from build123d import *

# Parameters (mm, degrees)
SKETCH1_W           = 95
SKETCH1_H           = 65
BOSS_EXTRUDE1_DEPTH = 5
FILLET2_R           = 4
SKETCH3_W           = 89.4
SKETCH3_H           = 59.4
BOSS_EXTRUDE3_DEPTH = 3
FILLET3_R           = 4
SHELL1_START        = -3
SHELL1_DEPTH        = 5.5


# Read off the part's stored shape, not the designer's step: Shell1
with BuildPart() as part:
    # Sketch1 → Boss-Extrude1 (new body)
    with BuildSketch(Plane(origin=(0, 0, 0), x_dir=(1, 0, 0), z_dir=(0, 1, 0))):
        with Locations((47.5, 32.5)):
            Rectangle(SKETCH1_W, SKETCH1_H)
    extrude(amount=BOSS_EXTRUDE1_DEPTH)

    # Fillet2
    fillet2_edges = [part.edges().sort_by_distance(p)[0] for p in [
        (95, 5, -32.5),
        (47.5, 5, -65),
        (0, 5, -32.5),
        (0, 2.5, -65),
        (95, 2.5, -65),
        (95, 2.5, 0),
        (0, 2.5, 0),
        (47.5, 5, 0),
    ]]
    fillet(fillet2_edges, radius=FILLET2_R)

    # Sketch3 → Boss-Extrude3 (add)
    with BuildSketch(Plane.XZ):
        with Locations((47.5, -32.5)):
            Rectangle(SKETCH3_W, SKETCH3_H)
    extrude(amount=BOSS_EXTRUDE3_DEPTH)

    # Fillet3
    fillet3_edges = [part.edges().sort_by_distance(p)[0] for p in [
        (2.8, -1.5, -2.8),
        (2.8, -1.5, -62.2),
        (92.2, -1.5, -62.2),
        (92.2, -1.5, -2.8),
    ]]
    fillet(fillet3_edges, radius=FILLET3_R)

    # Shell1 outline → Shell1 (cut)
    with BuildSketch(Plane(origin=(0, 0, 0), x_dir=(1, 0, 0), z_dir=(0, 1, 0)).offset(SHELL1_START)):
        with BuildLine():
            Line((5.3, 58.2), (5.3, 6.8))
            ThreePointArc((5.3, 6.8), (5.739339828, 5.739339828), (6.8, 5.3))
            Line((6.8, 5.3), (88.2, 5.3))
            ThreePointArc((88.2, 5.3), (89.260660172, 5.739339828), (89.7, 6.8))
            Line((89.7, 6.8), (89.7, 58.2))
            ThreePointArc((89.7, 58.2), (89.260660172, 59.260660172), (88.2, 59.7))
            Line((88.2, 59.7), (6.8, 59.7))
            ThreePointArc((6.8, 59.7), (5.739339828, 59.260660172), (5.3, 58.2))
        make_face()
    extrude(amount=SHELL1_DEPTH, mode=Mode.SUBTRACT)


solid = part.part
Verification items for the finished model (mm, model axes). A direction names the side the tool comes from. Round coordinates to 2 decimals unless told otherwise and drop trailing zeros. Order: outer loops, then holes, each group sorted by start corner. A loop starts at its lowest first (then second) coordinate and runs counter-clockwise, first axis right, second up.
1. Thickness scan on L1, parallel to Z at x = 57, y = 0.5; L2, parallel to X at y = -1.25, z = -47; L3, parallel to X at y = 0.75, z = -51.5. Record the ranges inside material, lowest first.
Final values:
L1: z = -65 to -59.7, -5.3 to 0
L2: x = 2.8 to 5.3, 89.7 to 92.2
L3: x = 0 to 5.3, 89.7 to 95
2. Section check A-A on x = 70. Record the cut outline in (y, z).
Final values:
outline: (-3, -62.2) - (0, -62.2) - (0, -65) - (1, -65) arc R4 ccw to (5, -61) - (5, -4) arc R4 ccw to (1, 0) - (0, 0) - (0, -2.8) - (-3, -2.8) - (-3, -5.3) - (2.5, -5.3) - (2.5, -59.7) - (-3, -59.7) - close
3. Go/stop test with flat-tipped pins: P1, Ø4, axis at x = 48, z = -30.5, coming from the -Y side; P2, Ø2.5, axis at y = -2, z = -22, coming from the +X side; P3, Ø1.5, axis at y = -1.5, z = -20, coming from the -X side. Record where each tip stops, or that it passes through.
Final values:
P1: stops at y = 2.5
P2: stops at x = 92.2
P3: stops at x = 2.8
4. Access from +Z, -Z, +X, -X, +Y, -Y to the whole of each face (thin tool, end or side, straight path). Record for faces 1 (the flat face through (47, -1, -2.8)), 2 (the flat face through (5.3, 0, -33)), 3 (the cylindrical face through (90.997, -1.521, -3.941)).
Final values:
face 1: +Z, +X, -X, -Y
face 2: -Y
face 3: +Z, +X, -Y
5. Section check C-C on z = -42.5. Record the cut outline in (x, y).
Final values:
outline: (0, 0) - (2.8, 0) - (2.8, -3) - (5.3, -3) - (5.3, 2.5) - (89.7, 2.5) - (89.7, -3) - (92.2, -3) - (92.2, 0) - (95, 0) - (95, 1) arc R4 ccw to (91, 5) - (4, 5) arc R4 ccw to (0, 1) - close
6. Section check B-B on y = -1.75. Record the cut outline in (x, z), then the cut area to 3 significant figures.
Final values:
outline: (2.8, -58.2) arc R4 ccw to (6.8, -62.2) - (88.2, -62.2) arc R4 ccw to (92.2, -58.2) - (92.2, -6.8) arc R4 ccw to (88.2, -2.8) - (6.8, -2.8) arc R4 ccw to (2.8, -6.8) - close; hole (5.3, -58.2) arc R1.5 ccw to (6.8, -59.7) - (88.2, -59.7) arc R1.5 ccw to (89.7, -58.2) - (89.7, -6.8) arc R1.5 ccw to (88.2, -5.3) - (6.8, -5.3) arc R1.5 ccw to (5.3, -6.8) - close
area: 707 mm2
